Job drawing, mm, ordinate dimensions from the low corner. One solid piece. A direction names the side the tool comes from. Give positions to 0.01 mm unless a question says otherwise; leave off trailing zeros. Write each loop counter-clockwise with the first axis right and the second up, starting at its lowest first coordinate (ties: lowest second). Pieces come first, ordered by that corner, then holes. Notation, with made-up numbers: (-22.75, 60) -> (27.25, 60) arc R21 ccw to (27.25, 95) -> close; hole circle Ø5 at (20.25, 21). An arc over 180 degrees is marked (long way). One line per question, with ' | ' between items. Start each with the question number.
(1) Tool access for the marked faces 5, 6, 7 and 8: list every direction of +Z, -Z, +X, -X, +Y, -Y with a clear straight run to the whole face (end or side of a thin tool).
(2) Band-saw the part on D-D, the plane y = 8.25. Give the cut face in (x, z).
(3) Band-saw the part on C-C, the plane y = 14. Give the cut face in (x, z).
(4) Pin check, flat tips, straight feed: P1, Ø1, axis at x = 44, y = 3.5, coming from the -Z side; P2, Ø3.5, axis at x = 27, z = 13.5, coming from the +Y side; P3, Ø4, axis at y = 10.5, z = 2, coming from the +X side. Stop position of each tip, or through.
(5) Drill centre lines: probe 1 along Y at (x, z) = (24, 18.5); probe 2 along Z at (x, y) = (45.5, 6.75); probe 3 along X at (y, z) = (4, 3.75). Where is each one in solid material? Low to high. Write a range as from..to.
(6) Pull direction Z, two halves, no side cores. Call the marked faces 1, 2, 3 and 4: released by +Z, released by -Z, zero draft, split by the parting line, or undercut.
(7) Band-saw the part on A-A, the plane x = 4. Give the cut face in (y, z), and give its area (3 significant figures).
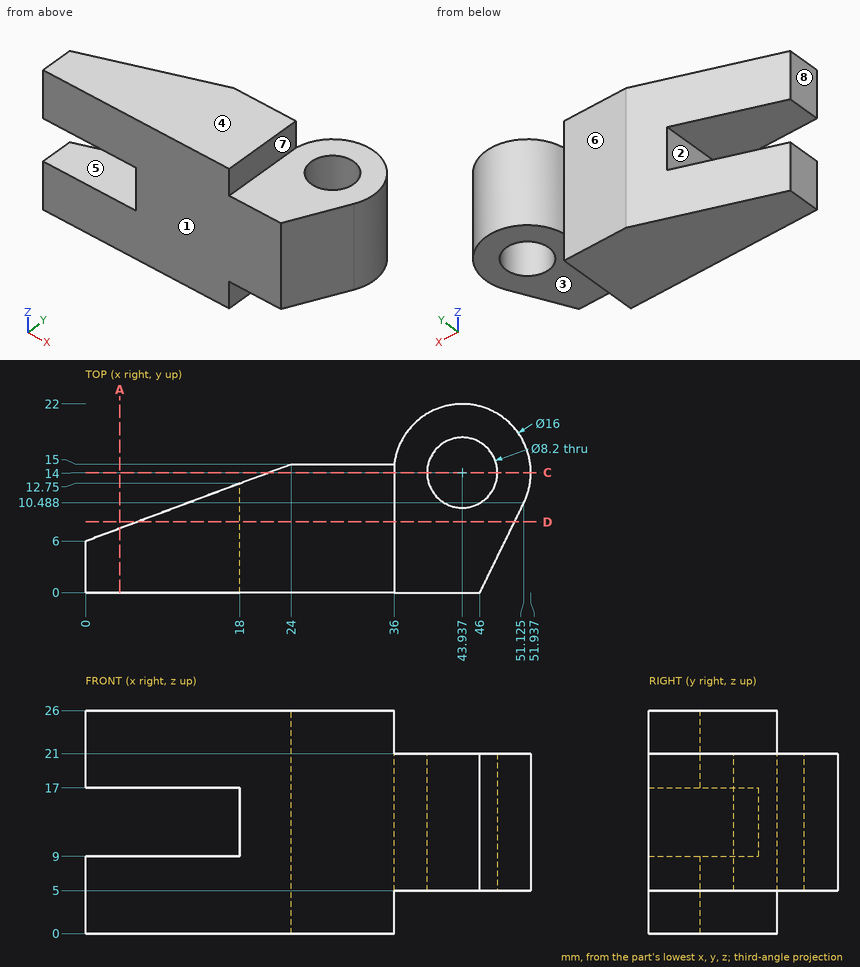
Results:
1) face 5: -X, +Y, -Y | face 6: +Z, -Z, -X, +Y | face 7: +Z, +X, +Y, -Y | face 8: +Z, -Z, -X, +Y, -Y
2) outline: (6, 0) -> (36, 0) -> (36, 5) -> (50.03, 5) -> (50.03, 21) -> (36, 21) -> (36, 26) -> (6, 26) -> (6, 17) -> (18, 17) -> (18, 9) -> (6, 9) -> close
3) outline: (21.33, 0) -> (36, 0) -> (36, 5) -> (39.84, 5) -> (39.84, 21) -> (36, 21) -> (36, 26) -> (21.33, 26) -> close; (48.04, 5) -> (51.94, 5) -> (51.94, 21) -> (48.04, 21) -> close
4) P1: stops at z = 5 | P2: stops at y = 15 | P3: stops at x = 36
5) probe 1: y = 0..15 | probe 2: z = 5..21 | probe 3: x = 0..36
6) face 1: zero draft | face 2: undercut | face 3: released by -Z | face 4: released by +Z
7) outline: (0, 0) -> (7.5, 0) -> (7.5, 9) -> (0, 9) -> close; (0, 17) -> (7.5, 17) -> (7.5, 26) -> (0, 26) -> close | area: 135 mm²
